```python
from build123d import *

# Parameters (mm, degrees)
F0_W     = 22.3
F0_H     = 1.5
F1_DEPTH = 42.3
F2_W     = 22.3
F2_H     = 1.5
F3_DEPTH = 42.3


with BuildPart() as f1:
    # F0 (on Front) → F1 (new body)
    with BuildSketch(Plane.XZ):
        with BuildLine():
            Line((-18, -10), (-20, -10))
            ThreePointArc((-20, -10), (-10, -20), (0, -10))
            Line((0, -10), (-2, -10))
            ThreePointArc((-2, -10), (-10, -18), (-18, -10))
        make_face()
        with BuildLine():
            Line((-20, -1.5), (-20, -10))
            ThreePointArc((-20, -10), (-17.0710678119, -2.9289321881), (-10, 0))
            Line((-10, 0), (-20, 0))
            Line((-20, 0), (-20, -1.5))
        make_face()
        with BuildLine():
            ThreePointArc((-10, 0), (-17.0710678119, -2.9289321881), (-20, -10))
            Line((-20, -10), (-18, -10))
            ThreePointArc((-18, -10), (-10, -2), (-2, -10))
            Line((-2, -10), (0, -10))
            ThreePointArc((0, -10), (-2.9289321881, -2.9289321881), (-10, 0))
        make_face()
        with BuildLine():
            ThreePointArc((-10, 0), (-2.9289321881, -2.9289321881), (0, -10))
            Line((0, -10), (0, 0))
            Line((0, 0), (-10, 0))
        make_face()
        with Locations((-31.15, -0.75)):
            Rectangle(F0_W, F0_H)
    extrude(amount=F1_DEPTH)

    # F2 (on Right) → F3 (join)
    with BuildSketch(Plane.YZ):
        with BuildLine():
            Line((0, 10), (-2, 10))
            ThreePointArc((-2, 10), (-10, 2), (-18, 10))
            Line((-18, 10), (-20, 10))
            ThreePointArc((-20, 10), (-17.0710678119, 2.9289321881), (-10, 0))
            ThreePointArc((-10, 0), (-2.9289321881, 2.9289321881), (0, 10))
        make_face()
        with BuildLine():
            ThreePointArc((-18, 10), (-10, 18), (-2, 10))
            Line((-2, 10), (0, 10))
            ThreePointArc((0, 10), (-10, 20), (-20, 10))
            Line((-20, 10), (-18, 10))
        make_face()
        with BuildLine():
            Line((0, 0), (0, 10))
            ThreePointArc((0, 10), (-2.9289321881, 2.9289321881), (-10, 0))
            Line((-10, 0), (0, 0))
        make_face()
        with BuildLine():
            ThreePointArc((-10, 0), (-17.0710678119, 2.9289321881), (-20, 10))
            Line((-20, 10), (-20, 1.5))
            Line((-20, 1.5), (-20, 0))
            Line((-20, 0), (-10, 0))
        make_face()
        with Locations((-31.15, 0.75)):
            Rectangle(F2_W, F2_H)
    extrude(amount=-F3_DEPTH)


solid = f1.part
```
Geometry check sheet. Reference: the model listing, model coordinates, mm. A direction names the side the tool comes from. Coordinates: 2 decimals unless noted, no trailing zeros. Order: outer loops, then holes, each group sorted by start corner. A loop starts at its lowest first (then second) coordinate and runs counter-clockwise, first axis right, second up. Notation, with made-up numbers: (29, -34.75) - (49, -34.75) arc R16 ccw to (49, -28.75) - close; hole circle Ø7 at (89, 58). An arc over 180 degrees is marked (long way). Use one line per item in the form item = value.
1. Gauge pin test, flat ends, axial feed: pin 1 (12 mm diameter, centred on x = -26.5, z = -5.5, fed in from +Y); pin 2 (2 mm diameter, centred on x = -30.5, y = -15, fed in from -Z); pin 3 (7 mm diameter, centred on x = -31, z = 6, fed in from -Y); pin 4 (1.5 mm diameter, centred on y = -24.5, z = -12, fed in from -X). Record the tip position at first contact, or that the pin passes through.
Here are the results:
pin_1 = 0
pin_2 = -1.5
pin_3 = -20
pin_4 = -19.92
2. Section check A-A (x = -10). Record the boundary of the cut face in (y, z), then the cut area to 3 significant figures.
Here are the results:
outline = (-42.3, -20) - (0, -20) - (0, -18) - (-42.3, -18) - close; (-42.3, -2) - (0, -2) - (0, 10) arc R10 ccw to (-20, 10) - (-20, 1.5) - (-42.3, 1.5) - close; hole circle Ø16 at (-10, 10)
area = 359 mm²
3. Access from +Z, -Z, +X, -X, +Y, -Y to the whole of each face (thin tool, end or side, straight path). Record for faces 1 (the face through (-21, -20, 6)), 2 (the face through (-16.4, -42.3, -4.5)), 3 (the face through (-20, -21, -6)).
Here are the results:
face_1 = +Z, +X, -X, -Y
face_2 = +Z, -Z, +X, -X, -Y
face_3 = -Z, -X, +Y, -Y
4. Scan lines: line 1 (Z direction, x = -29, y = -10); line 2 (Z direction, x = -10, y = -16); line 3 (Z direction, x = -38.5, y = -29.5). Record each from-to range of solid material in increasing order.
Here are the results:
line_1 = -1.5 to 2, 18 to 20
line_2 = -20 to -18, -2 to 4.71, 15.29 to 18
line_3 = -1.5 to 1.5
5. Draft check along Z on faces 4 (the face through (-31, -21, -1.5)), 5 (the face through (-16, 0, 1)), 6 (the face through (-8.27, -20.85, -17.81)). Enter one of: pulls with the +Z half, pulls with the -Z half, needs draft (parallel to the pull), parting line crosses it, or undercut.
Here are the results:
face_4 = pulls with the -Z half
face_5 = needs draft
face_6 = undercut
6. Section check B-B (y = -10). Record the boundary of the cut face in (x, z).
Here are the results:
outline = (-42.3, -1.5) - (-20, -1.5) - (-20, -10) arc R10 ccw to (0, -10) - (0, 2) - (-42.3, 2) - close; (-42.3, 18) - (0, 18) - (0, 20) - (-42.3, 20) - close; hole circle Ø16 at (-10, -10)
7. Section check D-D (y = -24.5). Record the boundary of the cut face in (x, z), then the cut area to 3 significant figures.
Here are the results:
outline = (-42.3, -1.5) - (-20, -1.5) - (-20, -10) arc R10 ccw to (0, -10) - (0, 1.5) - (-42.3, 1.5) - close; hole circle Ø16 at (-10, -10)
area = 253 mm²
8. Section check C-C (z = 12). Record the boundary of the cut face in (x, y), then the cut area to 3 significant figures.
Here are the results:
outline = (-42.3, -19.8) - (0, -19.8) - (0, -17.75) - (-42.3, -17.75) - close; (-42.3, -2.25) - (0, -2.25) - (0, -0.2) - (-42.3, -0.2) - close
area = 174 mm²
